```python
from build123d import *

# Parameters (mm, degrees)
ESBO_O2_R                = 2
RESSALTO_EXTRUS_O1_DEPTH = 5.5
ESBO_O3_R                = 33.530734639
ESBO_O3_R_2              = 27
CORTE_EXTRUS_O1_DEPTH    = 11
ESBO_O4_R                = 3.25
CORTE_EXTRUS_O3_DEPTH    = 3.5
CORTE_EXTRUS_O4_DEPTH    = 205.13414707
PADR_OCIRCULAR7_COUNT    = 4


with BuildPart() as part:
    # Esboço1 → revolução (revolve)
    with BuildSketch(Plane.XY, mode=Mode.PRIVATE) as revolu_o_sk:
        with BuildLine():
            Line((-63.834530413, 0), (-63.834530413, 27))
            Line((-63.834530413, 27), (123.665469587, 27))
            Line((123.665469587, 27), (123.665469587, 36.5))
            Line((123.665469587, 36.5), (129.165469587, 36.5))
            Line((129.165469587, 36.5), (129.165469587, 24))
            Line((129.165469587, 24), (-55.834512047, 24))
            ThreePointArc((-55.834512047, 24), (-59.370057826, 22.535540399), (-60.834530413, 19))
            Line((-60.834530413, 19), (-60.834530413, 0))
            Line((-60.834530413, 0), (-63.834530413, 0))
        make_face()
    revolve(revolu_o_sk.sketch.rotate(Axis((-88.99, 0, 0), (1, 0, 0)), 90), axis=Axis((-88.99, 0, 0), (1, 0, 0)))

    # Esboço4 → Corte-extrusão3 (cut)
    with BuildSketch(Plane.ZY.offset(-123.665469587)):
        with Locations((0, 31.75)):
            Circle(ESBO_O4_R)
    corte_extrus_o3 = extrude(amount=-CORTE_EXTRUS_O3_DEPTH, mode=Mode.SUBTRACT)

    # Esboço4<3> → Corte-extrusão4 (cut, through all)
    with BuildSketch(Plane.ZY.offset(-123.665469587)):
        with BuildLine():
            ThreePointArc((0, 33.25), (-1.5, 31.75), (0, 30.25))
            Line((0, 30.25), (0, 33.25))
        make_face()
        with BuildLine():
            Line((0, 33.25), (0, 30.25))
            ThreePointArc((0, 30.25), (1.060660172, 30.689339828), (1.5, 31.75))
            ThreePointArc((1.5, 31.75), (1.060660172, 32.810660172), (0, 33.25))
        make_face()
    corte_extrus_o4 = extrude(amount=-CORTE_EXTRUS_O4_DEPTH, mode=Mode.SUBTRACT)

    # PadrãoCircular7: Corte-extrusão3, Corte-extrusão4 ×4 about axis
    padr_ocircular7_axis = Axis((0, 0, 0), (1, 0, 0))
    add([corte_extrus_o3.rotate(padr_ocircular7_axis, i * 360 / PADR_OCIRCULAR7_COUNT) for i in range(1, PADR_OCIRCULAR7_COUNT)], mode=Mode.SUBTRACT)
    add([corte_extrus_o4.rotate(padr_ocircular7_axis, i * 360 / PADR_OCIRCULAR7_COUNT) for i in range(1, PADR_OCIRCULAR7_COUNT)], mode=Mode.SUBTRACT)


with BuildPart() as body_2:
    # Esboço2 → Ressalto-extrusão1 (new, symmetric)
    with BuildSketch(Plane.XY):
        Polygon((-63.834530413, 27), (-73.834530413, 0), (-63.834530413, -27), align=None)
        with Locations((-68.834530413, 0)):
            Circle(ESBO_O2_R, mode=Mode.SUBTRACT)
    extrude(amount=RESSALTO_EXTRUS_O1_DEPTH, both=True)

    # Esboço3 → Corte-extrusão1 (cut)
    with BuildSketch(Plane.ZY.offset(63.834530413)):
        Circle(ESBO_O3_R)
        Circle(ESBO_O3_R_2, mode=Mode.SUBTRACT)
    extrude(amount=CORTE_EXTRUS_O1_DEPTH, mode=Mode.SUBTRACT)


with BuildPart() as part_1:
    add(part.part)

    # Combinar1: union body 2
    add(body_2.part)


solid = part_1.part
```
Geometry: final body of the model. Coordinates: model frame, mm. A direction names the side the tool comes from. Coordinates: 2 decimals unless noted, no trailing zeros. Order: outer loops, then holes, each group sorted by start corner. A loop starts at its lowest first (then second) coordinate and runs counter-clockwise, first axis right, second up. Notation, with made-up numbers: M 56,72.5 L 113,72.5 A7 ccw 113,76.5 Z; hole C 19,59 d3. An arc over 180 degrees is marked long. Answer in a Markdown table with one row per item. Add a question column.
Q1. Section query A-A on x = -29.5. Return the cut outline in (y, z).
Q2. Reachability of faces 4 (the cylindrical face through (-66.927, 0.601, -0.077)), 5 (the cylindrical face through (35.37, -7.21, 22.89)), 6 (the flat face through (-66.7, 0.4, -5.5)), 7 (the flat face through (-63.835, 0, 14)), 8 (the cylindrical face through (125.391, -0.705, -28.577)) from +Z, -Z, +X, -X, +Y, -Y: full face, straight path, thin tool, end or side. Return the list, or none.
Q3. Contact query for flat-ended pins moving along their axis: P1, Ø12, axis at x = -8.5, z = 25.5, coming from the -Y side; P2, Ø11, axis at y = 6, z = 17.5, coming from the -X side; P3, Ø5, axis at x = 21, z = -5, coming from the -Y side. Output: stop coordinate, or through.
Q4. Line query: L1, parallel to Y at x = 87.5, z = 0; L2, parallel to Y at x = 124.7, z = 0; L3, parallel to X at y = 24.5, z = -25. Output: solid intervals per line, ascending.
Q5. Mould query, pull axis Y, two halves, no side actions, for faces 1 (the flat face through (-63.835, 0, -14)), 2 (the flat face through (-68.765, 13.689, 0.077)), 3 (the flat face through (127.165, 30, 1)). Classes: released by +Y, released by -Y, zero draft, split by the parting line, or undercut.
Completed:
| question | item | result |
|---|---|---|
| 1 | outline | C 0,0 d54; hole C 0,0 d48 |
| 2 | face 4 | +Z, -Z |
| 2 | face 5 | +X |
| 2 | face 6 | -Z, -X, +Y, -Y |
| 2 | face 7 | +Z, -X, +Y, -Y |
| 2 | face 8 | -X |
| 3 | P1 | stops at y = -18.67 |
| 3 | P2 | stops at x = -63.83 |
| 3 | P3 | stops at y = -26.88 |
| 4 | L1 | y = -27 to -24, 24 to 27 |
| 4 | L2 | y = -36.5 to -35, -28.5 to -24, 24 to 28.5, 35 to 36.5 |
| 4 | L3 | x = 123.67 to 129.17 |
| 5 | face 1 | zero draft |
| 5 | face 2 | released by +Y |
| 5 | face 3 | undercut |
